Part model, mm, in its own coordinate system. Face numbers are marked on the shaded views. A direction names the side the tool comes from. Give positions to 0.01 mm unless a question says otherwise; leave off trailing zeros. Write each loop counter-clockwise with the first axis right and the second up, starting at its lowest first coordinate (ties: lowest second). Pieces come first, ordered by that corner, then holes. Notation, with made-up numbers: M -34,36 L 2,36 A28 ccw 2,73 Z; hole C -25,35.25 d2. An arc over 180 degrees is marked long. Use CSV: the item, a comma, the result in double quotes. Start each with the question number.
1. Band-saw the part on B-B, the plane x = -9.5. List the corners of the cut face in (y, z), then the cut area to 3 significant figures.
2. Drill centre lines: line 1 along Z through (x, y) = (-18.16, 1.05) (3 decimals); line 2 along Y through (x, z) = (14, -1.5); line 3 along Z through (x, y) = (8, 3.25). Where is each one in solid material? Low to high. Write a range as from..to.
3. Band-saw the part on D-D, the plane y = 5.5. List the corners of the cut face in (x, z).
4. Drop flat-ended pins along their axis: pin 1 Ø3.5 at (x, z) = (18.16, -21.205) entering from -Y; pin 2 Ø3.5 at (y, z) = (4.5, 17.5) entering from +X; pin 3 Ø2 at (x, z) = (-10.5, 1) entering from +Y; pin 4 Ø1.8 at (x, y) = (3.5, 4) entering from -Z. Give the stop position or say it passes through.
5. Band-saw the part on C-C, the plane z = -11. List the corners of the cut face in (x, y), then the cut area to 3 significant figures.
6. 3-axis set-ups, long thin cutter, end or side, ignore diameter. For the marked faces 1, 2 and 3: which of +Z, -Z, +X, -X, +Y, -Y reach the whole face in a straight line?
7. Band-saw the part on A-A, the plane x = 18.16. List the corners of the cut face in (y, z) (3 decimals), then the cut area to 3 significant figures.
from build123d import *

# Parameters (mm, degrees)
SKETCH1_W             = 41.4
SKETCH1_H             = 48.3
SKETCH1_R             = 1.5
BOSS_EXTRUDE1_DEPTH   = 1.6
SKETCH2_W             = 21
SKETCH2_H             = 7
BOSS_EXTRUDE2_DEPTH   = 8.85
CHAMFER1_SIZE         = 3
CHAMFER1_SIZE2        = 1.732050808
CHAMFER1_PART_2_SIZE  = 3
CHAMFER1_PART_2_SIZE2 = 1.732050808


with BuildPart() as part:
    # Sketch1 → Boss-Extrude1 (new body)
    with BuildSketch(Plane(origin=(0, 0, 0), x_dir=(1, 0, 0), z_dir=(0, 1, 0))):
        Rectangle(SKETCH1_W, SKETCH1_H)
        with Locations((-18.16, 21.205)):
            Circle(SKETCH1_R, mode=Mode.SUBTRACT)
        with Locations((18.16, 21.205)):
            Circle(SKETCH1_R, mode=Mode.SUBTRACT)
        with Locations((18.16, -21.205)):
            Circle(SKETCH1_R, mode=Mode.SUBTRACT)
        with Locations((-18.16, -21.205)):
            Circle(SKETCH1_R, mode=Mode.SUBTRACT)
    extrude(amount=BOSS_EXTRUDE1_DEPTH)

    # Sketch2 → Boss-Extrude2 (add)
    with BuildSketch(Plane(origin=(0, 1.6, 0), x_dir=(1, 0, 0), z_dir=(0, 1, 0))):
        with Locations((0, -17.35)):
            Rectangle(SKETCH2_W, SKETCH2_H)
    extrude(amount=BOSS_EXTRUDE2_DEPTH)

    # Chamfer1
    chamfer1_edges = [part.edges().sort_by_distance(p)[0] for p in [
        (0, 10.45, 13.85),
    ]]
    chamfer1_side = [part.faces().sort_by_distance(p)[0] for p in [
        (0, 6.025, 13.85),
    ]]
    chamfer(chamfer1_edges, length=CHAMFER1_SIZE, length2=CHAMFER1_SIZE2, reference=chamfer1_side[0])

    # Chamfer1 part 2
    chamfer1_part_2_edges = [part.edges().sort_by_distance(p)[0] for p in [
        (0, 10.45, 20.85),
    ]]
    chamfer1_part_2_side = [part.faces().sort_by_distance(p)[0] for p in [
        (0, 6.025, 20.85),
    ]]
    chamfer(chamfer1_part_2_edges, length=CHAMFER1_PART_2_SIZE, length2=CHAMFER1_PART_2_SIZE2, reference=chamfer1_part_2_side[0])


solid = part.part
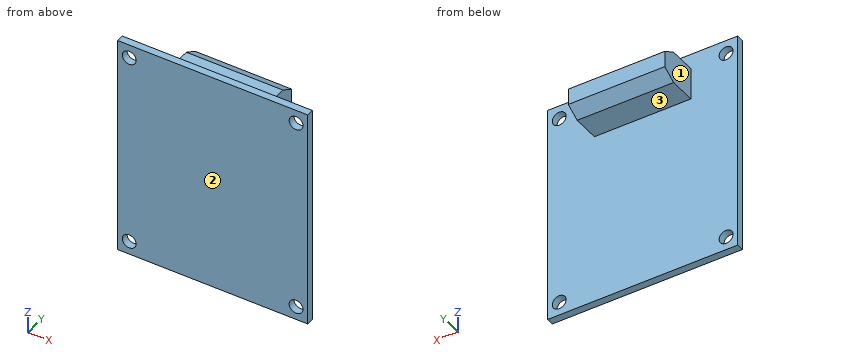
Output:
1,outline,"M 0,-24.15 L 1.6,-24.15 L 1.6,13.85 L 7.45,13.85 L 10.45,15.58 L 10.45,19.12 L 7.45,20.85 L 1.6,20.85 L 1.6,24.15 L 0,24.15 Z"
1,area,"134 mm²"
2,line 1,"z = -24.15..-22.705, -19.705..19.705, 22.705..24.15"
2,line 2,"y = 0..1.6"
2,line 3,"z = 13.85..20.85"
3,outline,"M -10.5,13.85 L 10.5,13.85 L 10.5,20.85 L -10.5,20.85 Z"
4,pin 1,"stops at y = 0"
4,pin 2,"stops at x = 10.5"
4,pin 3,"stops at y = 1.6"
4,pin 4,"stops at z = 13.85"
5,outline,"M -20.7,0 L 20.7,0 L 20.7,1.6 L -20.7,1.6 Z"
5,area,"66.2 mm²"
6,face 1,"+Z, -Z, -X, +Y"
6,face 2,"+Z, -Z, +X, -X, -Y"
6,face 3,"-Z, +X, -X, +Y"
7,outline,"M 0,-24.15 L 1.6,-24.15 L 1.6,-22.705 L 0,-22.705 Z; M 0,-19.705 L 1.6,-19.705 L 1.6,19.705 L 0,19.705 Z; M 0,22.705 L 1.6,22.705 L 1.6,24.15 L 0,24.15 Z"
7,area,"67.7 mm²"
